The listing builds one solid part. Answer for the finished solid, in the listing's coordinates (mm). Face numbers are marked on the shaded views. A direction names the side the tool comes from. Round coordinates to 2 decimals unless told otherwise and drop trailing zeros. Loops run counter-clockwise (first coordinate to the right, second up) from the corner with the lowest first, then second, coordinate; pieces in that order, holes last. Notation, with made-up numbers: (-26, -25) -> (-7, -25) arc R29 ccw to (-7, 5) -> close; hole circle Ø1 at (-19.5, -31). An arc over 180 degrees is marked (long way). One line per question, with ' | ' between items.
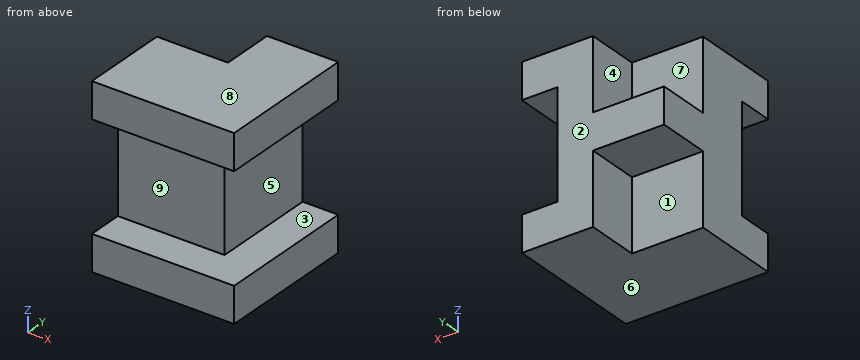
Autodesk Fusion 360 part; units mm, degrees
sketch "Sketch1" plane through (0, 0, 0) normal (0, 0, 1) x (1, 0, 0)
  line L0 (0, 0) -> (0, 25)
  line L1 (0, 25) -> (20, 25)
  line L2 (20, 25) -> (20, 40)
  line L3 (20, 40) -> (40, 40)
  line L4 (40, 40) -> (40, 0)
  line L5 (40, 0) -> (0, 0)
  dimension "d1" = 40
  dimension "d2" = 25
  dimension "d3" = 20
  dimension "d4" = 15
extrude "Extrude1" add sketch "Sketch1" along normal mid plane 50
sketch "Sketch2" plane through (0, 0, 0) normal (0, 0, 1) x (1, 0, 0)
  line L0 (0, 40) -> (20, 40)
  line L1 (20, 40) -> (20, 25)
  line L2 (20, 25) -> (0, 25)
  line L3 (0, 25) -> (0, 40)
  point P0 (20, 25)
  point P1 (0, 25)
  dimension "d7" = 20
  dimension "d8" = 15
extrude "Extrude2" add sketch "Sketch2" along normal mid plane 10
sketch "Sketch3" plane through (0, 40, 0) normal (0, 1, 0) x (-1, 0, 0)
  line L0 (-20, -25) -> (-20, -5)
  line L1 (-20, -5) -> (0, -5)
  line L2 (0, -5) -> (0, 5)
  line L3 (0, 5) -> (-20, 5)
  line L4 (-20, 5) -> (-20, 25)
  line L5 (-20, 25) -> (-40, 25)
  line L6 (-40, 25) -> (-40, -25)
  line L7 (-40, -25) -> (-20, -25)
  line L8 (-40, -15) -> (-30, -15)
  line L9 (-30, -15) -> (-30, 15)
  line L10 (-30, 15) -> (-40, 15)
  line L11 (-40, 15) -> (-40, -15)
  dimension "d11" = 10
  dimension "d12" = 10
  dimension "d13" = 30
  dimension "d14" = 10
extrude "Extrude3" cut sketch "Sketch3" against normal blind 85 contours L6 L8 L9 L10 L11
sketch "Sketch4" plane through (0, 0, 0) normal (1, 0, 0) x (0, 0, -1)
  line L0 (15, 0) -> (15, 10)
  line L1 (15, 10) -> (-15, 10)
  line L2 (-15, 10) -> (-15, 0)
  line L3 (25, 0) -> (-25, 0)
  dimension "d17" = 10
  dimension "d18" = 10
  dimension "d19" = 10
  dimension "d20" = 30
extrude "Extrude4" cut sketch "Sketch4" along normal blind 88
Q1. A cutting plane is placed at C-C on x = 15. Give the vertices of the cut face in (y, z).
Numbers:
outline: (0, -25) -> (25, -25) -> (25, -5) -> (40, -5) -> (40, 5) -> (25, 5) -> (25, 25) -> (0, 25) -> (0, 15) -> (10, 15) -> (10, -15) -> (0, -15) -> close
Q2. For the marked faces 1, 2, 3, 4 and 5, determine the directions among +Z, -Z, +X, -X, +Y, -Y from which every point of the face is accessible in a straight line to the end or side of a thin tool.
Numbers:
face 1: -Z, -X, +Y | face 2: +Z, -Z, +X, -X, +Y | face 3: +X, -Y | face 4: +Z, -X, +Y | face 5: +X, +Y, -Y
Q3. A cutting plane is placed at D-D on y = 23.5. Give the vertices of the cut face in (x, z).
Numbers:
outline: (0, -25) -> (40, -25) -> (40, -15) -> (30, -15) -> (30, 15) -> (40, 15) -> (40, 25) -> (0, 25) -> close
Q4. A cutting plane is placed at A-A on y = 6.5. Give the vertices of the cut face in (x, z).
Numbers:
outline: (0, -25) -> (40, -25) -> (40, -15) -> (0, -15) -> close; (0, 15) -> (40, 15) -> (40, 25) -> (0, 25) -> close
Q5. A cutting plane is placed at B-B on z = 8. Give the vertices of the cut face in (x, y), plus the area to 3 significant figures.
Numbers:
outline: (0, 10) -> (30, 10) -> (30, 40) -> (20, 40) -> (20, 25) -> (0, 25) -> close | area: 600 mm^2
Q6. For a pull along Z with two mould halves and no side action, classify the marked faces 6, 7, 8 and 9 as pulls with the +Z half, pulls with the -Z half, needs draft (parallel to the pull), parting line crosses it, or undercut.
Numbers:
face 6: pulls with the -Z half | face 7: needs draft | face 8: pulls with the +Z half | face 9: undercut
Q7. Given pin 1 Ø9 at (x, z) = (7.5, 1) entering from -Y; pin 2 Ø4 at (x, y) = (11.5, 36) entering from +Z; pin 3 Ø4.5 at (x, y) = (11.5, 29.5) entering from -Z, each flat-ended and moving along its own axis, determine where each tip first touches the part or whether it passes through.
Numbers:
pin 1: y = 10 | pin 2: z = 5 | pin 3: z = -5
Q8. Find the intervals of material crossed by line 1 (Z direction, x = 31, y = 10); line 2 (Y direction, x = 15, z = -6); line 3 (Z direction, x = 5, y = 30), in increasing order. Write a range as from..to.
Numbers:
line 1: -25..-15, 15..25 | line 2: 10..25 | line 3: -5..5
